Here's how the part is built. I have some questions about the finished solid (model axes, mm). A direction names the side the tool comes from. Coordinates: 2 decimals unless noted, no trailing zeros. Write each loop counter-clockwise with the first axis right and the second up, starting at its lowest first coordinate (ties: lowest second). Pieces come first, ordered by that corner, then holes. Notation, with made-up numbers: (23.25, -10) -> (40.25, -10) arc R19 ccw to (40.25, 1) -> close; hole circle Ø6 at (-21, 11). An arc over 180 degrees is marked (long way). Put each result on its own line as item: value.
```python
from build123d import *

# Parameters (mm, degrees)
F1_DEPTH = 45
F2_R     = 3.3
F3_DEPTH = 243.651


with BuildPart() as f1:
    # F0 (on Front) → F1 (new body, symmetric)
    with BuildSketch(Plane.XZ):
        Polygon((118.65, 13.4125), (118.65, 1.5875), (-118.65, 1.5875), (-118.65, 13.4125), (-121.825, 13.4125), (-121.825, 1.5875), (-121.825, -1.5875), (-118.65, -1.5875), (118.65, -1.5875), (121.825, -1.5875), (121.825, 1.5875), (121.825, 13.4125), align=None)
    extrude(amount=F1_DEPTH, both=True)

    # F2 (on face) → F3 (cut, through all)
    with BuildSketch(Plane.YZ.offset(121.825)):
        with Locations((-25, 8.4125)):
            Circle(F2_R)
        with Locations((25, 8.4125)):
            Circle(F2_R)
    extrude(amount=-F3_DEPTH, mode=Mode.SUBTRACT)


solid = f1.part
```
Item 1: Please list where these lines run through material, in increasing order: line 1 along X through (y, z) = (-8, 7.25) (3 decimals); line 2 along Z through (x, y) = (-120.45, -25). Write a range as from..to.
Output:
line 1: x = -121.825..-118.65, 118.65..121.825
line 2: z = -1.59..5.11, 11.71..13.41
Item 2: Imagine slicing it at A-A on y = -25. State how many separate pieces and enclosed holes the cut face has, then the cut area to 3 significant figures.
Output:
separate pieces: 3
enclosed holes: 0
area: 807 mm²
Item 3: Imagine slicing it at C-C on x = -34. Write out the boundary of the cut face in (y, z), then the cut area to 3 significant figures.
Output:
outline: (-45, -1.59) -> (45, -1.59) -> (45, 1.59) -> (-45, 1.59) -> close
area: 286 mm²
Item 4: Which directions (+Z, -Z, +X, -X, +Y, -Y) give clear straight access to the entire face, cutting with the end or side of a thin tool? Please do faces 1 (the flat face through (-1, 45, 0)), 2 (the flat face through (118.65, -1, 8)).
Output:
face 1: +Z, -Z, +X, -X, +Y
face 2: +Z, +Y, -Y
Item 5: If we mould it in two halves opening along Z, with no side actions, what happens to faces 3 (the flat face through (-121.825, -1, 6)), 4 (the cylindrical face through (-120.22, 28.05, 7.15)), 5 (the flat face through (2, -1, 1.588)), 6 (the cylindrical face through (120.26, -21.95, 7.15))? For each: released by +Z, released by -Z, zero draft, split by the parting line, or undercut.
Output:
face 3: zero draft
face 4: undercut
face 5: released by +Z
face 6: undercut
